Autodesk Inventor part; units mm, degrees
ref_plane "YZ Plane" through (0, 0, 0) normal (1, 0, 0) x (0, 1, 0)
ref_plane "XZ Plane" through (0, 0, 0) normal (0, 1, 0) x (-1, 0, 0)
ref_plane "XY Plane" through (0, 0, 0) normal (0, 0, 1) x (1, 0, 0)
sketch "Sketch1" plane through (0, 0, 0) normal (0, 1, 0) x (-1, 0, 0)
  circle A0 centre (0, 0) radius 2
  circle A1 centre (0, 0) radius 0.95
  circle A2 centre (-10.0688, 0.0006) radius 1.9997
  line L0 (-0.0618, -1.999) -> (-10.0688, -1.999)
  line L1 (-0.0618, 1.999) -> (-10.0686, 2.0003)
  circle A3 centre (-13.2373, 11.8352) radius 1.5
  line L2 (-8.0691, 0.0006) -> (-11.8022, 12.2717)
  line L3 (-12.0685, 0.0006) -> (-14.7373, 11.8352)
  circle A4 centre (-8.6896, 15.1639) radius 1
  line L4 (-13.2373, 13.3352) -> (-9.2441, 15.9961)
  line L5 (-13.2373, 10.3352) -> (-8.0733, 14.3764)
  dimension "d0" = 4
  dimension "d1" = 1.9
  dimension "d2" = 3
  dimension "d13" = 2
extrude "Extrusion1" add sketch "Sketch1" along normal blind 2 contours A0 | A0 L0 A2 L2 L1 | L2 A2 L1 | L1 A2 L3 A3 L5 L2 | A2 L2 | A2 L2 | L5 A3 L2 | A3 L5 L3 | A3 L5
sketch "Sketch2" plane through (0, 2, 0) normal (0, 1, 0) x (1, 0, 0)
  circle A0 centre (0, 0) radius 0.95
extrude "Extrusion2" add sketch "Sketch2" against normal blind 6 and the other way blind 0.5
thread "Thread1"
sketch "Sketch3" plane through (0, 2, 0) normal (0, 1, 0) x (1, 0, 0)
  circle A0 centre (0, 0) radius 1.8246
extrude "Extrusion3" add sketch "Sketch3" along normal blind 0.3
sketch "Sketch4" plane through (0, 2, 0) normal (0, 1, 0) x (1, 0, 0)
  circle A0 centre (7.388, -16.6186) radius 1
  arc A1 (11.8022, -12.2717) -> (14.7373, -11.8352) centre (13.2373, -11.8352) ccw
  line L0 (13.2373, -13.3352) -> (8.002, -17.4079)
  line L1 (8.6774, -2.0002) -> (11.8022, -12.2717)
  line L2 (11.6694, -11.8352) -> (6.7559, -15.8438)
  point P0 (0, 0)
  dimension "d14" = 2
extrude "Extrusion4" add sketch "Sketch4" against normal blind 2
properties part number "servo_hook"
Source: CAD feature listing. Evaluate the final solid. Frame: model axes, mm. A direction names the side the tool comes from. Round coordinates to 2 decimals unless told otherwise and drop trailing zeros. Loops run counter-clockwise (first coordinate to the right, second up) from the corner with the lowest first, then second, coordinate; pieces in that order, holes last. Notation, with made-up numbers: M 1,79 L 42,79 A23 ccw 42,89 Z; hole C 55.5,-5 d6. An arc over 180 degrees is marked long. Put each result on its own line as item: value.
(1) Section D-D, the plane x = 1.5. Return loops of the section in (y, z), and give its area (3 significant figures).
Solutions:
outline: M 0,-2 L 2,-2 L 2,-1.04 L 2.3,-1.04 L 2.3,1.04 L 2,1.04 L 2,2 L 0,2 Z
area: 8.62 mm²
(2) First-contact query: pin 1 (3 mm diameter, centred on x = 12.5, y = -0.5, fed in from -Z); pin 2 (4.5 mm diameter, centred on x = 8, z = 16, fed in from +Y); pin 3 (1.5 mm diameter, centred on y = -1.5, z = 4, fed in from -X); pin 4 (1 mm diameter, centred on x = 3.5, y = 1, fed in from +Z). Flat tips, straight axial feed; report the tip coordinate or a pass-through.
Solutions:
pin 1: z = -1.72
pin 2: y = 2
pin 3: through
pin 4: z = 2
(3) Access query for faces 1 (the face through (1, 2.3, 1)), 2 (the face through (-0.95, -1.97, -0.04)), 3 (the face through (10.152, 0.986, 6.849)). Directions: +Z, -Z, +X, -X, +Y, -Y. A direction counts if a zero-diameter tool reaches every point of the face in a straight line with its end or side. Return the directions, or none.
Solutions:
face 1: +Y
face 2: -Y
face 3: -X, +Y, -Y
(4) Section B-B, the plane y = 1. Return loops of the section in (x, z).
Solutions:
outline: M 0.06,-2 L 10.07,-2 A2 ccw 12.07,0 L 14.74,11.84 A1.5 ccw 13.24,13.34 L 8,17.41 A1 ccw 6.76,15.84 L 11.67,11.84 L 8.68,2 L 0.06,2 A2 ccw long Z
(5) Section C-C, the plane z = -0.25. Return loops of the section in (x, y), and give its area (3 significant figures).
Solutions:
outline: M -1.98,0 L -0.92,0 L -0.92,-4 L 0.92,-4 L 0.92,0 L 12.05,0 L 12.05,2 L 1.81,2 L 1.81,2.3 L 0.92,2.3 L 0.92,2.5 L -0.92,2.5 L -0.92,2.3 L -1.81,2.3 L -1.81,2 L -1.98,2 Z
area: 36.9 mm²
(6) Section A-A, the plane x = 9. Return loops of the section in (y, z).
Solutions:
outline: M 0,-2 L 2,-2 L 2,3.06 L 0,3.06 Z; M 0,14.01 L 2,14.01 L 2,16.63 L 0,16.63 Z
(7) Ray query, line 1 (Y direction, x = 10, z = 2); line 2 (Z direction, x = 0.75, y = 1); line 3 (X direction, y = 1, z = 9.75). Return the intervals inside material, ascending. Write a range as [from, to].
Solutions:
line 1: [0, 2]
line 2: [-2, 2]
line 3: [11.04, 14.27]
